Check sheet for the drawn part. Datum: minimum x, y, z corner. Units: mm. A direction names the side the tool comes from. Round coordinates to 2 decimals unless told otherwise and drop trailing zeros. Order: outer loops, then holes, each group sorted by start corner. A loop starts at its lowest first (then second) coordinate and runs counter-clockwise, first axis right, second up.
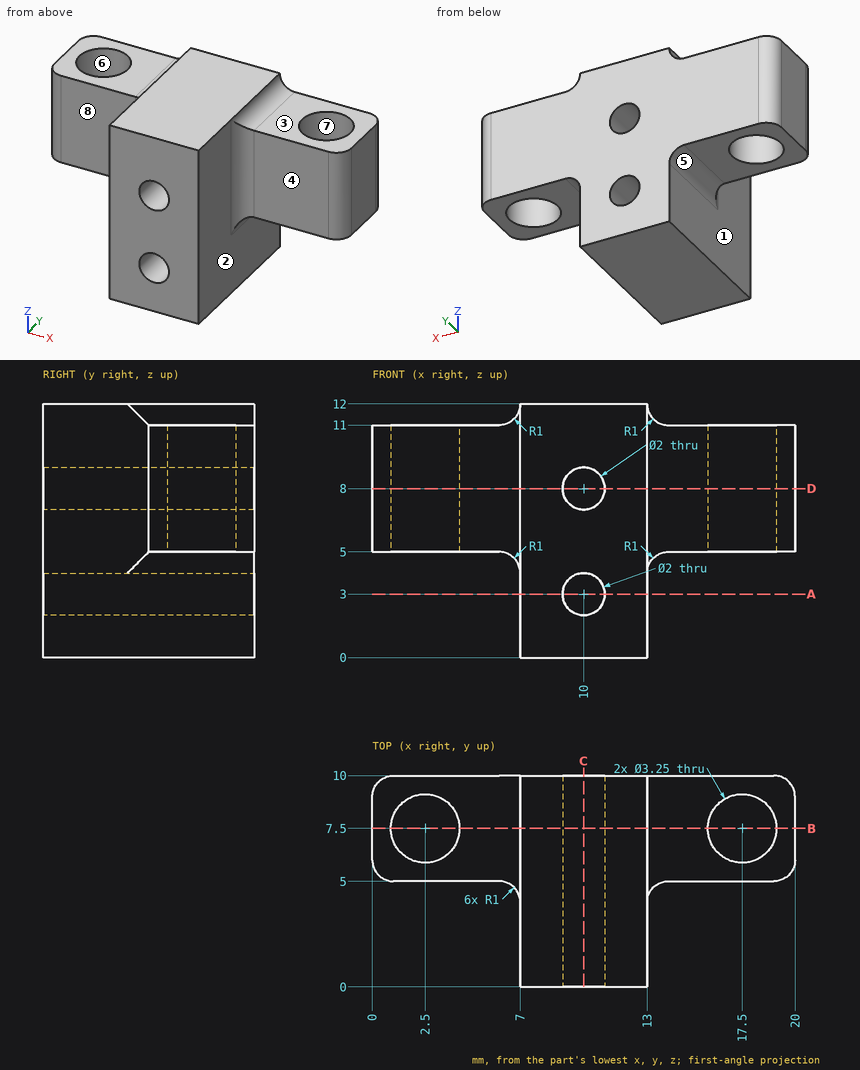
(1) Set-up check for the marked faces 1, 2, 3 and 4: record each of +Z, -Z, +X, -X, +Y, -Y from which the full face is reachable in a straight line by a thin tool's end or side.
Returned:
face 1: -Z, -X, -Y
face 2: -Z, +X, -Y
face 3: +Z, +X, +Y, -Y
face 4: +Z, -Z, +X, -Y
(2) Depth check by flat-ended pin: P1, Ø3, axis at x = 2.5, y = 7.5, coming from the -Z side; P2, Ø2.5, axis at x = 4.5, y = 8, coming from the +Z side; P3, Ø4, axis at x = 1.5, y = 7, coming from the -Z side; P4, Ø1.5, axis at x = 16.5, z = 7.5, coming from the -Y side. Enter the tip coordinate at first touch or a pass-through.
Returned:
P1: passes through
P2: stops at z = 11
P3: stops at z = 5
P4: stops at y = 5
(3) Sectioned sample at D-D, the plane z = 8. Record the cut outline in (x, y) (3 decimals).
Returned:
outline: (0, 6) arc R1 ccw to (1, 5) - (6, 5) arc R1 cw to (7, 4) - (7, 0) - (9, 0) - (9, 10) - (1, 10) arc R1 ccw to (0, 9) - close; (11, 0) - (13, 0) - (13, 4) arc R1 cw to (14, 5) - (19, 5) arc R1 ccw to (20, 6) - (20, 9) arc R1 ccw to (19, 10) - (11, 10) - close; hole circle Ø3.25 at (2.5, 7.5); hole circle Ø3.25 at (17.5, 7.5)
(4) Draft check along X on the marked faces 5, 6, 7 and 8. Enter one of: released by +X, released by -X, zero draft, split by the parting line, or undercut.
Returned:
face 5: released by -X
face 6: undercut
face 7: undercut
face 8: zero draft
(5) Material ranges on line 1 (Z direction, x = 10, y = 4.5); line 2 (Y direction, x = 2.5, z = 6.2) (3 decimals); line 3 (X direction, y = 8.5, z = 8.75), recorded low to high.
Returned:
line 1: z = 0 to 2, 4 to 7, 9 to 12
line 2: y = 5 to 5.875, 9.125 to 10
line 3: x = 0 to 1.22, 3.78 to 9.34, 10.66 to 16.22, 18.78 to 20
(6) Sectioned sample at A-A, the plane z = 3. Record the cut outline in (x, y), and give its area (3 significant figures).
Returned:
outline: (7, 0) - (9, 0) - (9, 10) - (7, 10) - close; (11, 0) - (13, 0) - (13, 10) - (11, 10) - close
area: 40.0 mm2
(7) Sectioned sample at C-C, the plane x = 10. Record the cut outline in (y, z), and give its area (3 significant figures).
Returned:
outline: (0, 0) - (10, 0) - (10, 2) - (0, 2) - close; (0, 4) - (10, 4) - (10, 7) - (0, 7) - close; (0, 9) - (10, 9) - (10, 12) - (0, 12) - close
area: 80.0 mm2
(8) Sectioned sample at B-B, the plane y = 7.5. Give the number of separate pieces and of enclosed holes in the cut face, and give its area (3 significant figures).
Returned:
separate pieces: 3
enclosed holes: 2
area: 112 mm2
